from build123d import *

# Parameters (mm, degrees)
SKETCH1_R           = 2.25
BOSS_EXTRUDE1_DEPTH = 1.5875


with BuildPart() as part:
    # Sketch1 → Boss-Extrude1 (new body)
    with BuildSketch(Plane.XY):
        Polygon((-26.9875, 0), (0, 0), (-22.106865795, -15.479394076), (44.420276683, -110.49), (77.365930897, -110.49), (88.926357353, -127), (111.033223148, -127), (111.033223148, -111.520605924), (26.9875, 8.509126065), (26.9875, 152.4), (-26.9875, 152.4), align=None)
        with Locations((98.333223148, -120.65)):
            Circle(SKETCH1_R, mode=Mode.SUBTRACT)
        with Locations((-14.2875, 12.7)):
            Circle(SKETCH1_R, mode=Mode.SUBTRACT)
        with Locations((-14.2875, 139.7)):
            Circle(SKETCH1_R, mode=Mode.SUBTRACT)
        with Locations((14.2875, 139.7)):
            Circle(SKETCH1_R, mode=Mode.SUBTRACT)
        with Locations((14.2875, 12.7)):
            Circle(SKETCH1_R, mode=Mode.SUBTRACT)
        with Locations((78.77672996, -87.595333778)):
            Circle(SKETCH1_R, mode=Mode.SUBTRACT)
        with Locations((18.988055574, -2.208257628)):
            Circle(SKETCH1_R, mode=Mode.SUBTRACT)
        with Locations((55.369460295, -103.985280447)):
            Circle(SKETCH1_R, mode=Mode.SUBTRACT)
        with Locations((-4.419214091, -18.598204297)):
            Circle(SKETCH1_R, mode=Mode.SUBTRACT)
    extrude(amount=BOSS_EXTRUDE1_DEPTH)


solid = part.part
Geometry: final body of the model. Coordinates: model frame, mm. A direction names the side the tool comes from. Round coordinates to 2 decimals unless told otherwise and drop trailing zeros. Loops run counter-clockwise (first coordinate to the right, second up) from the corner with the lowest first, then second, coordinate; pieces in that order, holes last. Notation, with made-up numbers: (-38.75, 40) - (0.25, 40) arc R20 ccw to (0.25, 52) - close; hole circle Ø5 at (89, -4.75). An arc over 180 degrees is marked (long way). Write each question's results on one line, items separated by ' | '. Start each with the question number.
1) Line query: probe 1 along X at (y, z) = (139.7, 0.7); probe 2 along Y at (x, z) = (-14, 1.15); probe 3 along X at (y, z) = (81.5, 0.35). Output: solid intervals per line, ascending. Write a range as [from, to].
2) Access query for faces 1 (the face through (-10.9, -7.63, 0.78)), 2 (the face through (26, 15, 1.588)). Directions: +Z, -Z, +X, -X, +Y, -Y. A direction counts if a zero-diameter tool reaches every point of the face in a straight line with its end or side. Return the directions, or none.
3) Cut plane A-A on z = 0.6. Count the separate pieces of the cut face and the enclosed holes in it, then the cut area to 3 significant figures.
4) Cut plane C-C on x = 35.5. Return loops of the section in (y, z).
5) First-contact query: P1, Ø7, axis at x = 98.33, y = -120.65, coming from the -Z side; P2, Ø0.5, axis at x = -10.5, z = 1, coming from the -Y side; P3, Ø0.8, axis at y = 116, z = 1, coming from the +X side. Flat tips, straight axial feed; report the tip coordinate or a pass-through.
6) Cut plane B-B on y = 85. Return loops of the section in (x, z).
Verdict:
1) probe 1: x = [-26.99, -16.54], [-12.04, 12.04], [16.54, 26.99] | probe 2: y = [-27.06, -9.8], [0, 10.47], [14.93, 137.47], [141.93, 152.4] | probe 3: x = [-26.99, 26.99]
2) face 1: +Z, -Z, -X | face 2: +Z, +X, -X, +Y, -Y
3) separate pieces: 1 | enclosed holes: 9 | area: 15,600 mm2
4) outline: (-97.75, 0) - (-3.65, 0) - (-3.65, 1.59) - (-97.75, 1.59) - close
5) P1: stops at z = 0 | P2: stops at y = -32.41 | P3: stops at x = 26.99
6) outline: (-26.99, 0) - (26.99, 0) - (26.99, 1.59) - (-26.99, 1.59) - close
